Autodesk Fusion 360 part; units mm, degrees
sketch "Main Body" plane through (0, 0, 0) normal (0, 0, 1) x (1, 0, 0)
  line L0 (50.5, 21.5) -> (-50.5, 21.5)
  line L1 (-54.5, 17.5) -> (-54.5, -17.5)
  line L2 (-50.5, -21.5) -> (50.5, -21.5)
  line L3 (54.5, -17.5) -> (54.5, 17.5)
  arc A0 (-50.5, 21.5) -> (-54.5, 17.5) centre (-50.5, 17.5) ccw
  arc A1 (-54.5, -17.5) -> (-50.5, -21.5) centre (-50.5, -17.5) ccw
  arc A2 (50.5, -21.5) -> (54.5, -17.5) centre (50.5, -17.5) ccw
  arc A3 (54.5, 17.5) -> (50.5, 21.5) centre (50.5, 17.5) ccw
  line L4 (-54.5, 0) -> (54.5, 0) construction
  line L5 (0, 21.5) -> (0, -21.5) construction
  dimension "d3" = 4
  dimension "d4" = 4
  dimension "d5" = 4
  dimension "d6" = 4
  dimension "d7" = 109
  dimension "d8" = 43
extrude "Extrude1" add sketch "Main Body" along normal blind 1.6
sketch "Screw Holes" plane through (0, 0, 1.6) normal (0, 0, 1) x (-1, 0, 0)
  arc A0 (-54.5, -17.5) -> (-50.5, -21.5) centre (-50.5, -17.5) ccw
  line L0 (-50.5, -21.5) -> (50.5, -21.5)
  arc A1 (50.5, -21.5) -> (54.5, -17.5) centre (50.5, -17.5) ccw
  line L1 (54.5, -17.5) -> (54.5, 17.5)
  arc A2 (54.5, 17.5) -> (50.5, 21.5) centre (50.5, 17.5) ccw
  line L2 (50.5, 21.5) -> (-50.5, 21.5)
  arc A3 (-50.5, 21.5) -> (-54.5, 17.5) centre (-50.5, 17.5) ccw
  line L3 (-54.5, 17.5) -> (-54.5, -17.5)
  circle A4 centre (-51, 18) radius 1.19
  line L4 (51, 0) -> (-51, 0) construction
  line L5 (0, -18) -> (0, 18) construction
  line L6 (-51, -18) -> (-51, 18) construction
  line L7 (51, -18) -> (51, 18) construction
  circle A5 centre (-51, -18) radius 1.19
  circle A6 centre (0, 18) radius 1.19
  circle A7 centre (0, -18) radius 1.19
  circle A8 centre (51, -18) radius 1.19
  circle A9 centre (51, 18) radius 1.19
  dimension "d11" = 2.38
  dimension "d12" = 102
  dimension "d13" = 36
  dimension "d14" = 36
  dimension "d15" = 36
  dimension "d16" = 2.38
  dimension "d17" = 2.38
  dimension "d18" = 2.38
  dimension "d19" = 2.38
  dimension "d20" = 2.38
extrude "Extrude2" cut sketch "Screw Holes" against normal blind 1.6 contours A4 | A5 | A6 | A7 | A8 | A9
sketch "Button Holes" plane through (0, 0, 1.6) normal (0, 0, 1) x (-1, 0, 0)
  circle A0 centre (0, 18) radius 1.19
  circle A1 centre (0, -18) radius 1.19
  circle A2 centre (51, -18) radius 1.19
  circle A3 centre (-51, 18) radius 1.19
  circle A4 centre (-51, -18) radius 1.19
  circle A5 centre (51, 18) radius 1.19
  arc A6 (-54.5, -17.5) -> (-50.5, -21.5) centre (-50.5, -17.5) ccw
  line L0 (-50.5, -21.5) -> (50.5, -21.5)
  arc A7 (50.5, -21.5) -> (54.5, -17.5) centre (50.5, -17.5) ccw
  line L1 (54.5, -17.5) -> (54.5, 17.5)
  arc A8 (54.5, 17.5) -> (50.5, 21.5) centre (50.5, 17.5) ccw
  line L2 (50.5, 21.5) -> (-50.5, 21.5)
  arc A9 (-50.5, 21.5) -> (-54.5, 17.5) centre (-50.5, 17.5) ccw
  line L3 (-54.5, 17.5) -> (-54.5, -17.5)
  line L4 (-42.65, 0.05) -> (-42.65, 10.05) construction
  circle A10 centre (-42.65, 0.05) radius 1.75
  circle A11 centre (-42.65, 10.05) radius 1.75
  line L5 (0, 0) -> (-42.65, 0) construction
  line L6 (-42.65, 0) -> (-42.65, 0.05)
  dimension "d23" = 10
  dimension "d24" = 3.5
  dimension "d25" = 3.5
  dimension "d26" = 42.65
  dimension "d27" = 0.05
extrude "Extrude3" cut sketch "Button Holes" against normal blind 1.6 contours A10 | A11
sketch "Power Jack Hole" plane through (0, 0, 1.6) normal (0, 0, 1) x (-1, 0, 0)
  circle A0 centre (-42.65, 0.05) radius 1.75
  circle A1 centre (-42.65, 10.05) radius 1.75
  circle A2 centre (0, 18) radius 1.19
  circle A3 centre (0, -18) radius 1.19
  circle A4 centre (51, -18) radius 1.19
  circle A5 centre (-51, 18) radius 1.19
  circle A6 centre (-51, -18) radius 1.19
  circle A7 centre (51, 18) radius 1.19
  arc A8 (-54.5, -17.5) -> (-50.5, -21.5) centre (-50.5, -17.5) ccw
  line L0 (-50.5, -21.5) -> (50.5, -21.5)
  arc A9 (50.5, -21.5) -> (54.5, -17.5) centre (50.5, -17.5) ccw
  line L1 (54.5, -17.5) -> (54.5, 17.5)
  arc A10 (54.5, 17.5) -> (50.5, 21.5) centre (50.5, 17.5) ccw
  line L2 (50.5, 21.5) -> (-50.5, 21.5)
  arc A11 (-50.5, 21.5) -> (-54.5, 17.5) centre (-50.5, 17.5) ccw
  line L3 (-54.5, 17.5) -> (-54.5, -17.5)
  line L4 (0, 0) -> (41.3, 0) construction
  line L5 (41.3, 0) -> (41.3, 8.7) construction
  circle A12 centre (41.3, 8.7) radius 4.05
  dimension "d30" = 41.3
  dimension "d31" = 8.7
  dimension "d32" = 8.1
extrude "Extrude4" cut sketch "Power Jack Hole" against normal blind 1.6 contours A12
Verification items for the finished model (mm, model axes). Round coordinates to 2 decimals unless told otherwise and drop trailing zeros. Order: outer loops, then holes, each group sorted by start corner. A loop starts at its lowest first (then second) coordinate and runs counter-clockwise, first axis right, second up. Notation, with made-up numbers: (52, 66.5) -> (81, 66.5) arc R22 ccw to (81, 93.5) -> close; hole circle Ø11 at (43, 77). An arc over 180 degrees is marked (long way). Put each result on its own line as item: value. Start each with the question number.
(1) Draft check along Y on faces 1 (the face through (51.26, 19.16, 0.81)), 2 (the face through (-53.359, 20.297, 0.789)), 3 (the face through (53.359, -20.297, 0.789)). Enter one of: +Y half, -Y half, draft (parallel to the pull), parting line (faces both ways), or undercut.
(2) Section check B-B (z = 0.95). State how many separate pieces and enclosed holes the cut face has, then the cut area to 3 significant figures.
(3) Section check D-D (y = -10.05). Enter the section's corners in (x, z), then the cut area to 3 significant figures.
(4) Material ranges on line 1 along Y through (x, z) = (0, 1.1); line 2 along X through (y, z) = (-8.7, 1); line 3 along X through (y, z) = (19, 1.1), recorded low to high.
(5) Section check C-C (x = -38.5). Enter the section's corners in (y, z).
(6) Section check A-A (y = -0.05). Enter the section's corners in (x, z).
(7) Depth check by flat-ended pin: pin 1 Ø4 at (x, y) = (42.65, -0.05) entering from -Z. Enter the tip coordinate at first touch or a pass-through.
Completed:
1. face 1: undercut
1. face 2: +Y half
1. face 3: -Y half
2. separate pieces: 1
2. enclosed holes: 9
2. area: 4,580 mm2
3. outline: (-54.5, 0) -> (-45.12, 0) -> (-45.12, 1.6) -> (-54.5, 1.6) -> close; (-37.48, 0) -> (40.9, 0) -> (40.9, 1.6) -> (-37.48, 1.6) -> close; (44.4, 0) -> (54.5, 0) -> (54.5, 1.6) -> (44.4, 1.6) -> close
3. area: 157 mm2
4. line 1: y = -21.5 to -19.19, -16.81 to 16.81, 19.19 to 21.5
4. line 2: x = -54.5 to -45.35, -37.25 to 41.54, 43.76 to 54.5
4. line 3: x = -54.21 to -51.65, -50.35 to -0.65, 0.65 to 50.35, 51.65 to 54.21
5. outline: (-21.5, 0) -> (-11.63, 0) -> (-11.63, 1.6) -> (-21.5, 1.6) -> close; (-5.77, 0) -> (21.5, 0) -> (21.5, 1.6) -> (-5.77, 1.6) -> close
6. outline: (-54.5, 0) -> (40.9, 0) -> (40.9, 1.6) -> (-54.5, 1.6) -> close; (44.4, 0) -> (54.5, 0) -> (54.5, 1.6) -> (44.4, 1.6) -> close
7. pin 1: stops at z = 0
